from build123d import *

# Parameters (mm, degrees)
SKETCH1_W           = 90
SKETCH1_H           = 28
BOSS_EXTRUDE1_DEPTH = 2
SKETCH2_R           = 1.5
SKETCH2_W           = 78
SKETCH2_H           = 3
CUT_EXTRUDE1_DEPTH  = 95.276189995


with BuildPart() as part:
    # Sketch1 → Boss-Extrude1 (new body)
    with BuildSketch(Plane(origin=(0, 0, 0), x_dir=(1, 0, 0), z_dir=(0, 1, 0))):
        with Locations((45, 14)):
            Rectangle(SKETCH1_W, SKETCH1_H)
    extrude(amount=BOSS_EXTRUDE1_DEPTH)

    # Sketch2 → Cut-Extrude1 (cut, through all)
    with BuildSketch(Plane(origin=(0, 2, 0), x_dir=(1, 0, 0), z_dir=(0, 1, 0))):
        with Locations(Location((3, 23, 0), (0, 0, 270))):
            Circle(SKETCH2_R)
        with Locations(Location((3, 5, 0), (0, 0, 270))):
            Circle(SKETCH2_R)
        with Locations(Location((87, 23, 0), (0, 0, 270))):
            Circle(SKETCH2_R)
        with Locations(Location((87, 5, 0), (0, 0, 270))):
            Circle(SKETCH2_R)
        with Locations((45, 14)):
            Rectangle(SKETCH2_W, SKETCH2_H)
        with Locations((45, 5)):
            Rectangle(SKETCH2_W, SKETCH2_H)
        with Locations((45, 23)):
            Rectangle(SKETCH2_W, SKETCH2_H)
    extrude(amount=-CUT_EXTRUDE1_DEPTH, mode=Mode.SUBTRACT)


solid = part.part
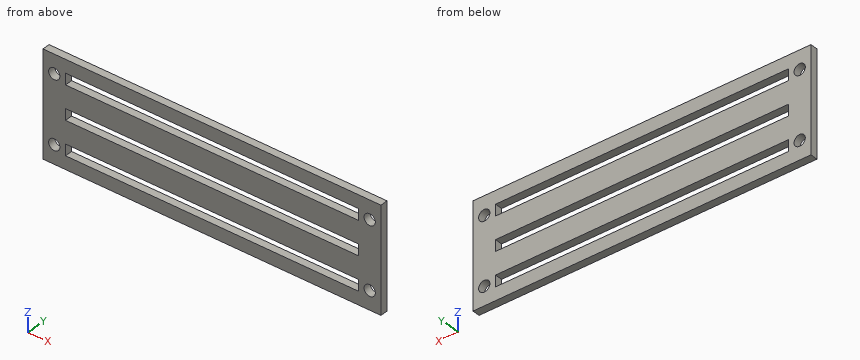
Input: part model. Units: mm. Frame: model coordinates. Give positions to 0.01 mm unless a question says otherwise; leave off trailing zeros. Loops run counter-clockwise (first coordinate to the right, second up) from the corner with the lowest first, then second, coordinate; pieces in that order, holes last. Notation, with made-up numbers: (-19, 44.25) -> (27, 44.25) arc R17 cw to (27, 75.25) -> close; hole circle Ø10 at (-29, 67.25). An arc over 180 degrees is marked (long way). Answer as a JSON object with one key per item and string values. Group by question number.
Item 1: Cut plane A-A, the plane z = -13.75. Return the cut outline in (x, y).
Item 2: Line query: probe 1 along Z at (x, y) = (87, 1.1); probe 2 along Z at (x, y) = (50.5, 0.3); probe 3 along X at (y, z) = (0.45, -23). Output: solid intervals per line, ascending.
Item 3: Cut plane C-C, the plane y = 1.15. Return the cut outline in (x, z), and give its area (3 significant figures).
Item 4: Cut plane B-B, the plane x = 66. Return the cut outline in (y, z).
Item 5: Cut plane D-D, the plane x = 3. Return the cut outline in (y, z), and give its area (3 significant figures).
Checks:
{
 "1": {"outline": "(0, 0) -> (6, 0) -> (6, 2) -> (0, 2) -> close; (84, 0) -> (90, 0) -> (90, 2) -> (84, 2) -> close"},
 "2": {"probe 1": "z = -28 to -24.5, -21.5 to -6.5, -3.5 to 0", "probe 2": "z = -28 to -24.5, -21.5 to -15.5, -12.5 to -6.5, -3.5 to 0", "probe 3": "x = 0 to 1.5, 4.5 to 6, 84 to 85.5, 88.5 to 90"},
 "3": {"outline": "(0, -28) -> (90, -28) -> (90, 0) -> (0, 0) -> close; hole circle Ø3 at (3, -23); hole circle Ø3 at (3, -5); hole (6, -24.5) -> (84, -24.5) -> (84, -21.5) -> (6, -21.5) -> close; hole (6, -15.5) -> (84, -15.5) -> (84, -12.5) -> (6, -12.5) -> close; hole (6, -6.5) -> (84, -6.5) -> (84, -3.5) -> (6, -3.5) -> close; hole circle Ø3 at (87, -23); hole circle Ø3 at (87, -5)", "area": "1,790 mm²"},
 "4": {"outline": "(0, -28) -> (2, -28) -> (2, -24.5) -> (0, -24.5) -> close; (0, -21.5) -> (2, -21.5) -> (2, -15.5) -> (0, -15.5) -> close; (0, -12.5) -> (2, -12.5) -> (2, -6.5) -> (0, -6.5) -> close; (0, -3.5) -> (2, -3.5) -> (2, 0) -> (0, 0) -> close"},
 "5": {"outline": "(0, -28) -> (2, -28) -> (2, -24.5) -> (0, -24.5) -> close; (0, -21.5) -> (2, -21.5) -> (2, -6.5) -> (0, -6.5) -> close; (0, -3.5) -> (2, -3.5) -> (2, 0) -> (0, 0) -> close", "area": "44.0 mm²"}
}
